```python
from build123d import *

# Parameters (mm, degrees)
SKETCH1_R           = 15.53845
BOSS_EXTRUDE1_DEPTH = 8.6741
SKETCH2_R           = 22.0726
BOSS_EXTRUDE2_DEPTH = 1.4097
SKETCH3_R           = 19.2151
BOSS_EXTRUDE3_DEPTH = 6.9977
BOSS_EXTRUDE5_START = 8.4074
SKETCH2_3_R         = 22.0726
BOSS_EXTRUDE5_DEPTH = 1.2954
SKETCH5_R           = 3.1877
CUT_EXTRUDE1_DEPTH  = 37.223056126


with BuildPart() as part:
    # Sketch1 → Boss-Extrude1 (new body)
    with BuildSketch(Plane.XY):
        Circle(SKETCH1_R)
    extrude(amount=-BOSS_EXTRUDE1_DEPTH)

    # Sketch2 → Boss-Extrude2 (add)
    with BuildSketch(Plane.XY):
        Circle(SKETCH2_R)
    extrude(amount=BOSS_EXTRUDE2_DEPTH)

    # Sketch3 → Boss-Extrude3 (add)
    with BuildSketch(Plane.XY.offset(1.4097)):
        Circle(SKETCH3_R)
    extrude(amount=BOSS_EXTRUDE3_DEPTH)

    # Sketch2<3> → Boss-Extrude5 (add)
    with BuildSketch(Plane.XY.offset(BOSS_EXTRUDE5_START)):
        Circle(SKETCH2_3_R)
    extrude(amount=BOSS_EXTRUDE5_DEPTH)

    # Sketch5 → Cut-Extrude1 (cut, through all)
    with BuildSketch(Plane(origin=(0, 0, -8.6741), x_dir=(-1, 0, 0), z_dir=(0, 0, -1))):
        Circle(SKETCH5_R)
    extrude(amount=-CUT_EXTRUDE1_DEPTH, mode=Mode.SUBTRACT)


solid = part.part
```
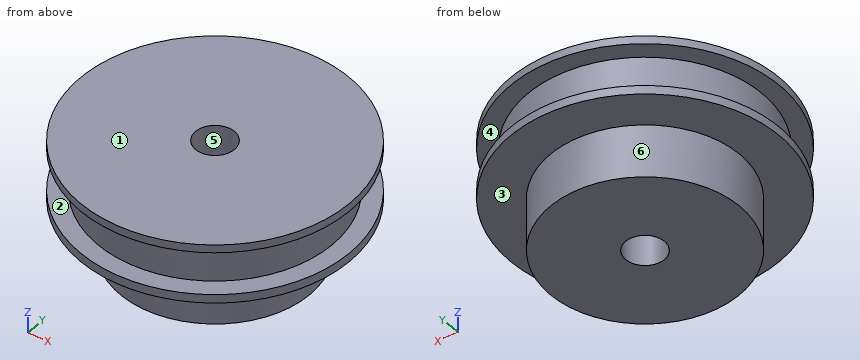
The listing builds one solid part. Answer for the finished solid, in the listing's coordinates (mm). Face numbers are marked on the shaded views. A direction names the side the tool comes from. Coordinates: 2 decimals unless noted, no trailing zeros. Loops run counter-clockwise (first coordinate to the right, second up) from the corner with the lowest first, then second, coordinate; pieces in that order, holes last. Notation, with made-up numbers: (-24, 61) - (31, 61) arc R17 ccw to (31, 82) - close; hole circle Ø2 at (8.25, 54.25). An arc over 180 degrees is marked (long way). Use a Markdown table: item, result. Add a question column.
1) Find the intervals of material crossed by line 1 (Y direction, x = 0, z = -0.25); line 2 (Y direction, x = 0, z = 2.5); line 3 (Z direction, x = -19, y = 6), in increasing order.
2) For the marked faces 1, 2 and 3, determine the directions among +Z, -Z, +X, -X, +Y, -Y from which every point of the face is accessible in a straight line to the end or side of a thin tool.
3) The part is cut by section D-D, the plane y = 13. Give the vertices of the cut face in (x, z).
4) Given pin 1 (1 mm diameter, centred on x = -15, z = 5, fed in from -Y); pin 2 (5 mm diameter, centred on x = -11.5, z = 7.5, fed in from -Y), each flat-ended and moving along its own axis, determine where each tip first touches the part or whether it passes through.
5) The mould has two halves that part along Y. Classify the marked faces 4, 5 and 6: released by +Y, released by -Y, zero draft, split by the parting line, or undercut.
6) The part is cut by section A-A, the plane y = 0. Give the vertices of the cut face in (x, z), and give its area (3 significant figures).
7) The part is cut by section C-C, the plane z = 3. Give the vertices of the cut face in (x, y), and give its area (3 significant figures).
Here are the results:
| question | item | result |
|---|---|---|
| 1 | line 1 | y = -15.54 to -3.19, 3.19 to 15.54 |
| 1 | line 2 | y = -19.22 to -3.19, 3.19 to 19.22 |
| 1 | line 3 | z = 0 to 1.41, 8.41 to 9.7 |
| 2 | face 1 | +Z, +X, -X, +Y, -Y |
| 2 | face 2 | none |
| 2 | face 3 | -Z |
| 3 | outline | (-17.84, 0) - (-8.51, 0) - (-8.51, -8.67) - (8.51, -8.67) - (8.51, 0) - (17.84, 0) - (17.84, 1.41) - (14.15, 1.41) - (14.15, 8.41) - (17.84, 8.41) - (17.84, 9.7) - (-17.84, 9.7) - (-17.84, 8.41) - (-14.15, 8.41) - (-14.15, 1.41) - (-17.84, 1.41) - close |
| 4 | pin 1 | stops at y = -12.61 |
| 4 | pin 2 | stops at y = -20.08 |
| 5 | face 4 | zero draft |
| 5 | face 5 | undercut |
| 5 | face 6 | split by the parting line |
| 6 | outline | (-22.07, 0) - (-15.54, 0) - (-15.54, -8.67) - (-3.19, -8.67) - (-3.19, 9.7) - (-22.07, 9.7) - (-22.07, 8.41) - (-19.22, 8.41) - (-19.22, 1.41) - (-22.07, 1.41) - close; (3.19, -8.67) - (15.54, -8.67) - (15.54, 0) - (22.07, 0) - (22.07, 1.41) - (19.22, 1.41) - (19.22, 8.41) - (22.07, 8.41) - (22.07, 9.7) - (3.19, 9.7) - close |
| 6 | area | 541 mm^2 |
| 7 | outline | circle Ø38.43 at (0, 0); hole circle Ø6.38 at (0, 0) |
| 7 | area | 1,130 mm^2 |
